```python
from build123d import *

# Parameters (mm, degrees)
SKETCH1_R           = 3
BOSS_EXTRUDE1_DEPTH = 3
SKETCH5_W           = 1
SKETCH5_H           = 15
SKETCH4_W           = 1
SKETCH4_H           = 15
SKETCH7_W           = 1
SKETCH7_H           = 15
SKETCH6_W           = 1
SKETCH6_H           = 15


with BuildPart() as part:
    # Sketch1 → Boss-Extrude1 (new body)
    with BuildSketch(Plane(origin=(0, 5.01, 0), x_dir=(1, 0, 0), z_dir=(0, 1, 0))):
        with BuildLine():
            Line((-7.5, -7.5), (-7.5, 7.5))
            Line((-7.5, 7.5), (-4, 15))
            ThreePointArc((-4, 15), (0, 19), (4, 15))
            Line((4, 15), (7.5, 7.5))
            Line((7.5, 7.5), (7.5, -7.5))
            Line((7.5, -7.5), (4, -15))
            ThreePointArc((4, -15), (0, -19), (-4, -15))
            Line((-4, -15), (-7.5, -7.5))
        make_face()
        with Locations((0, 15)):
            Circle(SKETCH1_R, mode=Mode.SUBTRACT)
        with Locations((0, -15)):
            Circle(SKETCH1_R, mode=Mode.SUBTRACT)
    boss_extrude1 = extrude(amount=BOSS_EXTRUDE1_DEPTH)

    # Sketch5 → Loft2 section 0
    with BuildSketch(Plane(origin=(0, 0, 0), x_dir=(1, 0, 0), z_dir=(0, 1, 0))):
        with Locations((7, 0)):
            Rectangle(SKETCH5_W, SKETCH5_H)
    # Sketch4 → Loft2 section 1
    with BuildSketch(Plane(origin=(0, 5.01, 0), x_dir=(1, 0, 0), z_dir=(0, 1, 0))):
        with Locations((7, 0)):
            Rectangle(SKETCH4_W, SKETCH4_H)
    loft2 = loft()

    # Sketch7 → Loft3 section 0
    with BuildSketch(Plane(origin=(0, 0, 0), x_dir=(1, 0, 0), z_dir=(0, 1, 0))):
        with Locations((-7, 0)):
            Rectangle(SKETCH7_W, SKETCH7_H)
    # Sketch6 → Loft3 section 1
    with BuildSketch(Plane(origin=(0, 5.01, 0), x_dir=(1, 0, 0), z_dir=(0, 1, 0))):
        with Locations((-7, 0)):
            Rectangle(SKETCH6_W, SKETCH6_H)
    loft3 = loft()

    # Mirror2: Boss-Extrude1, Loft2, Loft3 across plane
    add(boss_extrude1.mirror(Plane.ZX))
    add(loft2.mirror(Plane.ZX))
    add(loft3.mirror(Plane.ZX))


solid = part.part
```
Geometry check sheet. Reference: the model listing, model coordinates, mm. A direction names the side the tool comes from. Round coordinates to 2 decimals unless told otherwise and drop trailing zeros. Loops run counter-clockwise (first coordinate to the right, second up) from the corner with the lowest first, then second, coordinate; pieces in that order, holes last. Notation, with made-up numbers: M -7,-11 L 45,-11 A27 ccw 45,24 Z; hole C -39.5,54 d8. An arc over 180 degrees is marked long. Return JSON: item names as keys, results as strings. Group by question number.
(1) Set-up check for faces 4 (the face through (-7, 0, 7.5)), 5 (the face through (-7, 0, -7.5)), 6 (the face through (0, 8.01, 0)): record each of +Z, -Z, +X, -X, +Y, -Y from which the full face is reachable in a straight line by a thin tool's end or side.
(2) Section check D-D, the plane x = 6. Enter the section's corners in (y, z).
(3) Section check C-C, the plane z = 13.5. Enter the section's corners in (x, y).
(4) Section check A-A, the plane x = 0. Enter the section's corners in (y, z).
(5) Scan lines: line 1 along Z through (x, y) = (0, 6.75); line 2 along Y through (x, z) = (-1.5, 1); line 3 along X through (y, z) = (6.9, 15). Record each from-to range of solid material in increasing order. Write a range as [from, to].
(6) Mould release check, pull along X, two halves, no side actions. Record for faces 1 (the face through (-5.774, 6.489, -11.198)), 2 (the face through (-0.65, -6.49, 17.93)), 3 (the face through (0, 6, -19)): pulls with the +X half, pulls with the -X half, needs draft (parallel to the pull), parting line crosses it, or undercut.
(7) Section check B-B, the plane y = 4.5. Enter the section's corners in (x, z).
(8) Go/stop test with flat-tipped pins: pin 1 (0.5 mm diameter, centred on x = -7, y = 1.5, fed in from +Z); pin 2 (0.8 mm diameter, centred on x = -7, y = 1, fed in from -Z). Record where each tip stops, or that it passes through.
Data:
{
 "1": {"face 4": "+Z, +X, -X", "face 5": "-Z, +X, -X", "face 6": "+Z, -Z, +X, -X, +Y"},
 "2": {"outline": "M -8.01,-10.71 L -5.01,-10.71 L -5.01,10.71 L -8.01,10.71 Z; M 5.01,-10.71 L 8.01,-10.71 L 8.01,10.71 L 5.01,10.71 Z"},
 "3": {"outline": "M -4.7,-8.01 L -2.6,-8.01 L -2.6,-5.01 L -4.7,-5.01 Z; M -4.7,5.01 L -2.6,5.01 L -2.6,8.01 L -4.7,8.01 Z; M 2.6,-8.01 L 4.7,-8.01 L 4.7,-5.01 L 2.6,-5.01 Z; M 2.6,5.01 L 4.7,5.01 L 4.7,8.01 L 2.6,8.01 Z"},
 "4": {"outline": "M -8.01,-19 L -5.01,-19 L -5.01,-18 L -8.01,-18 Z; M -8.01,-12 L -5.01,-12 L -5.01,12 L -8.01,12 Z; M -8.01,18 L -5.01,18 L -5.01,19 L -8.01,19 Z; M 5.01,-19 L 8.01,-19 L 8.01,-18 L 5.01,-18 Z; M 5.01,-12 L 8.01,-12 L 8.01,12 L 5.01,12 Z; M 5.01,18 L 8.01,18 L 8.01,19 L 5.01,19 Z"},
 "5": {"line 1": "[-19, -18], [-12, 12], [18, 19]", "line 2": "[-8.01, -5.01], [5.01, 8.01]", "line 3": "[-4, -3], [3, 4]"},
 "6": {"face 1": "pulls with the -X half", "face 2": "undercut", "face 3": "parting line crosses it"},
 "7": {"outline": "M -7.5,-7.5 L -6.5,-7.5 L -6.5,7.5 L -7.5,7.5 Z; M 6.5,-7.5 L 7.5,-7.5 L 7.5,7.5 L 6.5,7.5 Z"},
 "8": {"pin 1": "z = 7.5", "pin 2": "z = -7.5"}
}
